```python
from build123d import *

# Parameters (mm, degrees)
SCHIZZO1_R                     = 2.5
SCHIZZO1_R_2                   = 1.4
ESTRUSIONE_ESTRUSIONE1_DEPTH   = 4
ESTRUSIONE_ESTRUSIONE1_2_DEPTH = 4
ESTRUSIONE_ESTRUSIONE1_3_DEPTH = 4
ESTRUSIONE_ESTRUSIONE1_4_DEPTH = 4
ESTRUSIONE_ESTRUSIONE2_DEPTH   = 8
SCHIZZO3_R                     = 2.25
TAGLIO_ESTRUSIONE1_DEPTH       = 18
SCHIZZO4_W                     = 10
SCHIZZO4_H                     = 8
TAGLIO_ESTRUSIONE2_DEPTH       = 7


with BuildPart() as part:
    # Schizzo1 → Estrusione-Estrusione1 (new body)
    with BuildSketch(Plane.XY):
        with Locations((-29.25, 24.5)):
            Circle(SCHIZZO1_R)
        with Locations((-29.25, 24.5)):
            Circle(SCHIZZO1_R_2, mode=Mode.SUBTRACT)
    extrude(amount=ESTRUSIONE_ESTRUSIONE1_DEPTH)



with BuildPart() as body_2:
    # Schizzo1 → Estrusione-Estrusione1 2 (new body)
    with BuildSketch(Plane.XY):
        with Locations((29.25, 24.5)):
            Circle(SCHIZZO1_R)
        with Locations((29.25, 24.5)):
            Circle(SCHIZZO1_R_2, mode=Mode.SUBTRACT)
    extrude(amount=ESTRUSIONE_ESTRUSIONE1_2_DEPTH)


with BuildPart() as body_3:
    # Schizzo1 → Estrusione-Estrusione1 3 (new body)
    with BuildSketch(Plane.XY):
        with Locations((29.25, -24.5)):
            Circle(SCHIZZO1_R)
        with Locations((29.25, -24.5)):
            Circle(SCHIZZO1_R_2, mode=Mode.SUBTRACT)
    extrude(amount=ESTRUSIONE_ESTRUSIONE1_3_DEPTH)


with BuildPart() as body_4:
    # Schizzo1 → Estrusione-Estrusione1 4 (new body)
    with BuildSketch(Plane.XY):
        with Locations((-29.25, -24.5)):
            Circle(SCHIZZO1_R)
        with Locations((-29.25, -24.5)):
            Circle(SCHIZZO1_R_2, mode=Mode.SUBTRACT)
    extrude(amount=ESTRUSIONE_ESTRUSIONE1_4_DEPTH)


with BuildPart() as part_1:
    add(part.part)

    add(body_2.part)  # Estrusione-Estrusione2 merges body 2

    add(body_3.part)  # Estrusione-Estrusione2 merges body 3

    add(body_4.part)  # Estrusione-Estrusione2 merges body 4
    # Schizzo2 → Estrusione-Estrusione2 (add)
    with BuildSketch(Plane.XY):
        Polygon((33.25, 27), (33.25, -28), (-33.25, -28), (-33.25, 27), (-24.75, 27), (-24.75, -13), (25.25, -13), (25.25, 27), align=None)
    extrude(amount=-ESTRUSIONE_ESTRUSIONE2_DEPTH)

    # Schizzo3 → Taglio-Estrusione1 (cut)
    with BuildSketch(Plane.XZ.offset(28)):
        with Locations((-15.75, -4)):
            Circle(SCHIZZO3_R)
        with Locations((20.25, -4)):
            Circle(SCHIZZO3_R)
    extrude(amount=-TAGLIO_ESTRUSIONE1_DEPTH, mode=Mode.SUBTRACT)

    # Schizzo4 → Taglio-Estrusione2 (cut)
    with BuildSketch(Plane.XZ.offset(28)):
        with Locations((-15.75, -4)):
            Rectangle(SCHIZZO4_W, SCHIZZO4_H)
        with Locations((20.25, -4)):
            Rectangle(SCHIZZO4_W, SCHIZZO4_H)
    extrude(amount=-TAGLIO_ESTRUSIONE2_DEPTH, mode=Mode.SUBTRACT)


solid = part_1.part
```
For this review, take the finished solid that the model builds, in its own axes (mm). A direction names the side the tool comes from. Give positions to 0.01 mm unless a question says otherwise; leave off trailing zeros. Loops run counter-clockwise (first coordinate to the right, second up) from the corner with the lowest first, then second, coordinate; pieces in that order, holes last. Notation, with made-up numbers: M -3,77.25 L 32,77.25 A19 cw 32,92.25 Z; hole C -32,38 d10. An arc over 180 degrees is marked long. One line per item, written item: value. Start each with the question number.
Q1. Machinability: for faces 1 (the face through (-13.67, -17.06, -4.86)), 2 (the face through (-29.553, -25.867, 1.972)), 3 (the face through (29, 27, -4)), 4 (the face through (0, -13, -4)), 5 (the face through (25.25, -25, -4)), which of the approach directions +Z, -Z, +X, -X, +Y, -Y give a long, thin tool a straight path to every point of the face, cutting with its end or side? Answer none if there is none.
Q2. Add section D-D (y = -24.5). Give the boundary of the cut face in (x, z).
Q3. Add section A-A (y = 24.5). Give the boundary of the cut face in (x, z).
Q4. Add section B-B (z = -4). Give the boundary of the cut face in (x, y).
Q5. Add section C-C (x = 20.25). Give the boundary of the cut face in (y, z).
Q6. Clearance check with flat-ended pins moving along their axes: pin 1 Ø4 at (x, z) = (-9.5, -6) entering from +Y; pin 2 Ø16.5 at (x, y) = (-1, -13) entering from +Z. State where each tip first meets the part, or that it passes through.
Q7. For L1, parallel to X at y = -25, z = -4; L2, parallel to Y at x = -29.25, z = 2.3; L3, parallel to Z at x = 20.25, y = -16.75, list the stretches that pass through material, from the lowest coordinate up.
Q8. Draft analysis for pull direction X (two halves, no side actions). For faces 6 (the face through (30, 23, 4)), 7 (the face through (22.396, -17.056, -3.324)), 8 (the face through (-29, -24, 0)), state which applies: released by +X, released by -X, zero draft, split by the parting line, or undercut.
Reply:
1. face 1: +Y, -Y
1. face 2: +Z
1. face 3: +Z, -Z, +X, -X, +Y
1. face 4: +Z, -Z, +Y
1. face 5: +Z, -Z, -Y
2. outline: M -33.25,-8 L -20.75,-8 L -20.75,0 L -26.75,0 L -26.75,4 L -27.85,4 L -27.85,0 L -30.65,0 L -30.65,4 L -31.75,4 L -31.75,0 L -33.25,0 Z; M -10.75,-8 L 15.25,-8 L 15.25,0 L -10.75,0 Z; M 25.25,-8 L 33.25,-8 L 33.25,0 L 31.75,0 L 31.75,4 L 30.65,4 L 30.65,0 L 27.85,0 L 27.85,4 L 26.75,4 L 26.75,0 L 25.25,0 Z
3. outline: M -33.25,-8 L -24.75,-8 L -24.75,0 L -26.75,0 L -26.75,4 L -27.85,4 L -27.85,0 L -30.65,0 L -30.65,4 L -31.75,4 L -31.75,0 L -33.25,0 Z; M 25.25,-8 L 33.25,-8 L 33.25,0 L 31.75,0 L 31.75,4 L 30.65,4 L 30.65,0 L 27.85,0 L 27.85,4 L 26.75,4 L 26.75,0 L 25.25,0 Z
4. outline: M -33.25,-28 L -20.75,-28 L -20.75,-21 L -18,-21 L -18,-13 L -24.75,-13 L -24.75,27 L -33.25,27 Z; M -13.5,-21 L -10.75,-21 L -10.75,-28 L 15.25,-28 L 15.25,-21 L 18,-21 L 18,-13 L -13.5,-13 Z; M 22.5,-21 L 25.25,-21 L 25.25,-28 L 33.25,-28 L 33.25,27 L 25.25,27 L 25.25,-13 L 22.5,-13 Z
5. outline: M -21,-8 L -13,-8 L -13,-6.25 L -21,-6.25 Z; M -21,-1.75 L -13,-1.75 L -13,0 L -21,0 Z
6. pin 1: y = -13
6. pin 2: z = 0
7. L1: -33.25 to -20.75, -10.75 to 15.25, 25.25 to 33.25
7. L2: -27 to -25.9, -23.1 to -22, 22 to 23.1, 25.9 to 27
7. L3: -8 to -6.25, -1.75 to 0
8. face 6: zero draft
8. face 7: undercut
8. face 8: undercut
